Verification items for the finished model (mm, model axes). A direction names the side the tool comes from. Give positions to 0.01 mm unless a question says otherwise; leave off trailing zeros. Order: outer loops, then holes, each group sorted by start corner. A loop starts at its lowest first (then second) coordinate and runs counter-clockwise, first axis right, second up. Notation, with made-up numbers: (-14.75, -20.75) -> (20.25, -20.75) arc R18 cw to (20.25, 10.25) -> close; hole circle Ø5 at (23, 79.5). An arc over 180 degrees is marked (long way). Write each question's results on one line, items separated by ' | '. Start each with the question number.
1. Cross-section at B-B, the plane x = 0. Enter the section's corners in (y, z).
2. Set-up check for faces 1 (the face through (22, 14, -10)), 2 (the face through (25.381, 18.126, -59.93)), 3 (the face through (-17, 28, -33)): record each of +Z, -Z, +X, -X, +Y, -Y from which the full face is reachable in a straight line by a thin tool's end or side.
3. Cross-section at A-A, the plane z = -32.5. Enter the section's corners in (x, y).
4. Cross-section at C-C, the plane y = 41. Enter the section's corners in (x, z).
5. Depth check by flat-ended pin: pin 1 Ø14 at (x, z) = (4, -60.5) entering from +Y; pin 2 Ø10 at (x, z) = (-15.5, -34) entering from +Y; pin 3 Ø1.5 at (y, z) = (22, -44) entering from +X; pin 4 Ø14.5 at (y, z) = (28.5, -22) entering from -X. Enter the tip coordinate at first touch or a pass-through.
6. Material ranges on L1, parallel to Z at x = -18.5, y = 23; L2, parallel to Y at x = -1, z = -32.5; L3, parallel to X at y = 31, z = -25.5, recorded low to high. Write a range as from..to.
7. Cross-section at D-D, the plane z = -15. Enter the section's corners in (x, y).
8. Mould release check, pull along Z, two halves, no side actions. Record for faces 4 (the face through (17, 28, -33)), 5 (the face through (0, 42, -56)), 6 (the face through (0, 17, -65)): +Z half, -Z half, draft (parallel to the pull), parting line (faces both ways), or undercut.
from build123d import *

# Parameters (mm, degrees)
BOSS_EXTRUDE1_DEPTH = 65
SKETCH2_R           = 15
BOSS_EXTRUDE2_DEPTH = 34
SKETCH3_R           = 9
CUT_EXTRUDE1_DEPTH  = 34
SKETCH4_W           = 45
SKETCH4_H           = 18
CUT_EXTRUDE2_DEPTH  = 17


with BuildPart() as part:
    # Sketch1 → Boss-Extrude1 (new body)
    with BuildSketch(Plane.XY):
        Polygon((-34, 0), (-34, 9), (-17, 27), (-17, 42), (17, 42), (17, 27), (34, 9), (34, 0), align=None)
    extrude(amount=-BOSS_EXTRUDE1_DEPTH)

    # Sketch2 → Boss-Extrude2 (add)
    with BuildSketch(Plane.ZY.offset(17)):
        with Locations((-32.5, 42)):
            Circle(SKETCH2_R)
    extrude(amount=-BOSS_EXTRUDE2_DEPTH)

    # Sketch3 → Cut-Extrude1 (cut)
    with BuildSketch(Plane.ZY.offset(17)):
        with Locations((-32.5, 42)):
            Circle(SKETCH3_R)
    extrude(amount=-CUT_EXTRUDE1_DEPTH, mode=Mode.SUBTRACT)

    # Sketch4 → Cut-Extrude2 (cut)
    with BuildSketch(Plane(origin=(-34, 0, 0), x_dir=(0, 0, -1), z_dir=(1, 0, 0))):
        with Locations((32.5, 18)):
            Rectangle(SKETCH4_W, SKETCH4_H)
    cut_extrude2 = extrude(amount=CUT_EXTRUDE2_DEPTH, mode=Mode.SUBTRACT)

    # Mirror1: Cut-Extrude2 across plane
    add(cut_extrude2.mirror(Plane(origin=(0, 0, 0), x_dir=(0, 0, 1), z_dir=(1, 0, 0))), mode=Mode.SUBTRACT)


solid = part.part
Results below:
1) outline: (0, -65) -> (42, -65) -> (42, -47.5) arc R15 ccw to (42, -17.5) -> (42, 0) -> (0, 0) -> close; hole circle Ø18 at (42, -32.5)
2) face 1: +X, +Y | face 2: +Z, -Z, +X, +Y | face 3: -X, +Y
3) outline: (-34, 0) -> (34, 0) -> (34, 9) -> (17, 9) -> (17, 33) -> (-17, 33) -> (-17, 9) -> (-34, 9) -> close; (-17, 51) -> (17, 51) -> (17, 57) -> (-17, 57) -> close
4) outline: (-17, -65) -> (17, -65) -> (17, -41.44) -> (-17, -41.44) -> close; (-17, -23.56) -> (17, -23.56) -> (17, 0) -> (-17, 0) -> close
5) pin 1: stops at y = 42 | pin 2: stops at y = 57 | pin 3: stops at x = 17 | pin 4: stops at x = -17
6) L1: z = -65..-55, -10..0 | L2: y = 0..33, 51..57 | L3: x = -17..17
7) outline: (-34, 0) -> (34, 0) -> (34, 9) -> (17, 9) -> (17, 42) -> (-17, 42) -> (-17, 9) -> (-34, 9) -> close
8) face 4: undercut | face 5: draft | face 6: -Z half
